```python
from build123d import *

# Parameters (mm, degrees)
SKETCH_1_R               = 275
SKETCH_1_R_2             = 255
EXTRUDE_1_DEPTH          = 10
EXTRUDE_2_DEPTH          = 10
SKETCH_8_R               = 2.65
SKETCH_8_R_2             = 1.65
SKETCH_8_R_3             = 2.15
CUT_EXTRUDE_1_DEPTH      = 21
SKETCH_9_OUTSIDE_W       = 707.614
SKETCH_9_OUTSIDE_H       = 707.614
CUT_EXTRUDE_2_DEPTH      = 21
EXTRUDE_3_DEPTH          = 10
SKETCH_11_W              = 11
SKETCH_11_H              = 6
CUT_EXTRUDE_3_DEPTH      = 509.636319812
CUT_EXTRUDE_3_DEPTH_BACK = 255.723154156
SKETCH_12_W              = 684.820669576
SKETCH_12_H              = 20
CUT_EXTRUDE_4_DEPTH      = 230.939436413
CUT_EXTRUDE_4_DEPTH_BACK = 534.420037555
SKETCH_14_R              = 4
CUT_EXTRUDE_6_DEPTH      = 11


with BuildPart() as part:
    # 草图1 → 凸台-拉伸1 (new body)
    with BuildSketch(Plane(origin=(0, 0, 0), x_dir=(1, 0, 0), z_dir=(0, 1, 0))):
        Circle(SKETCH_1_R)
        Circle(SKETCH_1_R_2, mode=Mode.SUBTRACT)
    extrude(amount=EXTRUDE_1_DEPTH)

    # 草图12 → 切除-拉伸4 (cut, two sides)
    with BuildSketch(Plane(origin=(84.710658728, 0, -125.893697679), x_dir=(-0.829665535, 0, -0.558260781), z_dir=(0.558260781, 0, -0.829665535))) as cut_extrude_4_sk:
        Rectangle(SKETCH_12_W, SKETCH_12_H)
    extrude(amount=CUT_EXTRUDE_4_DEPTH, mode=Mode.SUBTRACT)
    extrude(cut_extrude_4_sk.sketch, amount=-CUT_EXTRUDE_4_DEPTH_BACK, mode=Mode.SUBTRACT)


with BuildPart() as body_2:
    # 草图2 → 凸台-拉伸2 (new body)
    with BuildSketch(Plane(origin=(0, 10, 0), x_dir=(1, 0, 0), z_dir=(0, 1, 0))):
        with BuildLine():
            Line((-110.525139894, 257.262887824), (-25.423255477, 200))
            Line((-25.423255477, 200), (0, 200))
            Line((0, 200), (25.423255477, 200))
            Line((25.423255477, 200), (110.525139894, 257.262887824))
            ThreePointArc((110.525139894, 257.262887824), (197.989898732, 197.989898732), (257.262887824, 110.525139894))
            Line((257.262887824, 110.525139894), (200, 25.423255477))
            Line((200, 25.423255477), (200, 0))
            Line((200, 0), (200, -25.423255477))
            Line((200, -25.423255477), (257.262887824, -110.525139894))
            ThreePointArc((257.262887824, -110.525139894), (197.989898732, -197.989898732), (110.525139894, -257.262887824))
            Line((110.525139894, -257.262887824), (25.423255477, -200))
            Line((25.423255477, -200), (0, -200))
            Line((0, -200), (-25.423255477, -200))
            Line((-25.423255477, -200), (-110.525139894, -257.262887824))
            ThreePointArc((-110.525139894, -257.262887824), (-197.989898732, -197.989898732), (-257.262887824, -110.525139894))
            Line((-257.262887824, -110.525139894), (-200, -25.423255477))
            Line((-200, -25.423255477), (-200, 25.423255477))
            Line((-200, 25.423255477), (-257.262887824, 110.525139894))
            ThreePointArc((-257.262887824, 110.525139894), (-197.989898732, 197.989898732), (-110.525139894, 257.262887824))
        make_face()
        with BuildLine():
            Line((0, 185), (30, 185))
            Line((30, 185), (111.993839361, 240.171563565))
            ThreePointArc((111.993839361, 240.171563565), (187.383297014, 187.383297014), (240.171563565, 111.993839361))
            Line((240.171563565, 111.993839361), (185, 30))
            Line((185, 30), (185, 0))
            Line((185, 0), (185, -30))
            Line((185, -30), (240.171563565, -111.993839361))
            ThreePointArc((240.171563565, -111.993839361), (187.383297014, -187.383297014), (111.993839361, -240.171563565))
            Line((111.993839361, -240.171563565), (30, -185))
            Line((30, -185), (0, -185))
            Line((0, -185), (-30, -185))
            Line((-30, -185), (-111.993839361, -240.171563565))
            ThreePointArc((-111.993839361, -240.171563565), (-187.383297014, -187.383297014), (-240.171563565, -111.993839361))
            Line((-240.171563565, -111.993839361), (-185, -30))
            Line((-185, -30), (-185, 30))
            Line((-185, 30), (-240.171563565, 111.993839361))
            ThreePointArc((-240.171563565, 111.993839361), (-187.383297014, 187.383297014), (-111.993839361, 240.171563565))
            Line((-111.993839361, 240.171563565), (-30, 185))
            Line((-30, 185), (0, 185))
        make_face(mode=Mode.SUBTRACT)
    extrude(amount=EXTRUDE_2_DEPTH)

    # 草图8 → 切除-拉伸1 (cut, through all)
    with BuildSketch(Plane(origin=(0, 20, 0), x_dir=(1, 0, 0), z_dir=(0, 1, 0))):
        with Locations((-10, 192.5)):
            Circle(SKETCH_8_R)
        with Locations((10, 192.5)):
            Circle(SKETCH_8_R)
        with Locations((-10, -192.5)):
            Circle(SKETCH_8_R)
        with Locations((10, -192.5)):
            Circle(SKETCH_8_R)
        with Locations((192.5, 10)):
            Circle(SKETCH_8_R)
        with Locations((192.5, -10)):
            Circle(SKETCH_8_R)
        with Locations((-192.5, 10)):
            Circle(SKETCH_8_R)
        with Locations((-192.5, -10)):
            Circle(SKETCH_8_R)
        with Locations((-110.525139894, 248.223100485)):
            Circle(SKETCH_8_R_2)
        with Locations((-27.711627738, 192.5)):
            Circle(SKETCH_8_R)
        with Locations((-56.749921469, 212.03912734)):
            Circle(SKETCH_8_R)
        with Locations((-69.194904497, 220.413039057)):
            Circle(SKETCH_8_R)
        with Locations((-81.639887524, 228.786950774)):
            Circle(SKETCH_8_R)
        with Locations((-143.808163456, 231.45377032)):
            Circle(SKETCH_8_R_3)
        with Locations((-164.415519771, 217.299729706)):
            Circle(SKETCH_8_R_3)
        with Locations((-183.638937552, 201.316607082)):
            Circle(SKETCH_8_R_3)
        with Locations((-201.316607082, 183.638937552)):
            Circle(SKETCH_8_R_3)
        with Locations((-217.299729706, 164.415519771)):
            Circle(SKETCH_8_R_3)
        with Locations((-231.45377032, 143.808163456)):
            Circle(SKETCH_8_R_3)
        with Locations((-128.811575358, 240.123330241)):
            Circle(SKETCH_8_R)
        with Locations((-240.123330241, 128.811575358)):
            Circle(SKETCH_8_R)
        with Locations((-228.786950774, 81.639887524)):
            Circle(SKETCH_8_R)
        with Locations((-220.413039057, 69.194904497)):
            Circle(SKETCH_8_R)
        with Locations((-212.03912734, 56.749921469)):
            Circle(SKETCH_8_R)
        with Locations((-203.665215623, 44.304938442)):
            Circle(SKETCH_8_R)
        with Locations((-192.5, 27.711627738)):
            Circle(SKETCH_8_R)
        with Locations((-248.223100485, 110.525139894)):
            Circle(SKETCH_8_R_2)
        with Locations((192.5, 27.711627738)):
            Circle(SKETCH_8_R)
        with Locations((248.223100485, 110.525139894)):
            Circle(SKETCH_8_R_2)
        with Locations((203.665215623, 44.304938442)):
            Circle(SKETCH_8_R)
        with Locations((212.03912734, 56.749921469)):
            Circle(SKETCH_8_R)
        with Locations((220.413039057, 69.194904497)):
            Circle(SKETCH_8_R)
        with Locations((228.786950774, 81.639887524)):
            Circle(SKETCH_8_R)
        with Locations((240.123330241, 128.811575358)):
            Circle(SKETCH_8_R)
        with Locations((231.45377032, 143.808163456)):
            Circle(SKETCH_8_R_3)
        with Locations((128.811575358, 240.123330241)):
            Circle(SKETCH_8_R)
        with Locations((201.316607082, 183.638937552)):
            Circle(SKETCH_8_R_3)
        with Locations((183.638937552, 201.316607082)):
            Circle(SKETCH_8_R_3)
        with Locations((164.415519771, 217.299729706)):
            Circle(SKETCH_8_R_3)
        with Locations((143.808163456, 231.45377032)):
            Circle(SKETCH_8_R_3)
        with Locations((81.639887524, 228.786950774)):
            Circle(SKETCH_8_R)
        with Locations((69.194904497, 220.413039057)):
            Circle(SKETCH_8_R)
        with Locations((56.749921469, 212.03912734)):
            Circle(SKETCH_8_R)
        with Locations((110.525139894, 248.223100485)):
            Circle(SKETCH_8_R_2)
        with Locations((27.711627738, 192.5)):
            Circle(SKETCH_8_R)
        with Locations((217.299729706, 164.415519771)):
            Circle(SKETCH_8_R_3)
    extrude(amount=-CUT_EXTRUDE_1_DEPTH, mode=Mode.SUBTRACT)

    # 草图9 outside → 切除-拉伸2 (cut, through all)
    with BuildSketch(Plane(origin=(0, 20, 0), x_dir=(1, 0, 0), z_dir=(0, 1, 0))):
        Rectangle(SKETCH_9_OUTSIDE_W, SKETCH_9_OUTSIDE_H)
        Polygon((-28.994754224, 184.323595752), (-20.620842507, 196.76857878), (-83.675423179, 239.196398147), (-92.049334896, 226.751415119), align=None, mode=Mode.SUBTRACT)
    extrude(amount=-CUT_EXTRUDE_2_DEPTH, mode=Mode.SUBTRACT)

    # 草图10 → 凸台-拉伸3 (add)
    with BuildSketch(Plane(origin=(0, 20, 0), x_dir=(1, 0, 0), z_dir=(0, 1, 0))):
        Polygon((-28.539619055, 185), (-28.994754224, 184.323595752), (-30, 185), align=None)
    extrude(amount=-EXTRUDE_3_DEPTH)

    # 草图11 → 切除-拉伸3 (cut, two sides)
    with BuildSketch(Plane(origin=(-105.331501234, 0, -70.874881101), x_dir=(0.558260781, 0, -0.829665535), z_dir=(0.829665535, 0, 0.558260781))) as cut_extrude_3_sk:
        with Locations((144.240300571, 15)):
            Rectangle(SKETCH_11_W, SKETCH_11_H)
    extrude(amount=CUT_EXTRUDE_3_DEPTH, mode=Mode.SUBTRACT)
    extrude(cut_extrude_3_sk.sketch, amount=-CUT_EXTRUDE_3_DEPTH_BACK, mode=Mode.SUBTRACT)

    # 草图14 → 切除-拉伸6 (cut, through all)
    with BuildSketch(Plane.XZ.offset(-10)):
        with Locations((-47.5, -205.5)):
            Circle(SKETCH_14_R)
    extrude(amount=-CUT_EXTRUDE_6_DEPTH, mode=Mode.SUBTRACT)


solid = body_2.part
```
Input: part model. Units: mm. Frame: model coordinates. A direction names the side the tool comes from. Give positions to 0.01 mm unless a question says otherwise; leave off trailing zeros. Loops run counter-clockwise (first coordinate to the right, second up) from the corner with the lowest first, then second, coordinate; pieces in that order, holes last.
1) Section query C-C on x = -46. Return the cut outline in (y, z).
A:
outline: (10, -213.85) - (20, -213.85) - (20, -209.21) - (18, -209.21) - (18, -211.43) - (12, -211.43) - (12, -209.21) - (10, -209.21) - close; (10, -201.79) - (12, -201.79) - (12, -198.18) - (18, -198.18) - (18, -201.79) - (20, -201.79) - (20, -195.77) - (10, -195.77) - close
2) Section query D-D on z = -205.5. Return the cut outline in (x, y).
A:
outline: (-60.47, 10) - (-51.5, 10) - (-51.5, 12) - (-56.88, 12) - (-56.88, 18) - (-51.5, 18) - (-51.5, 20) - (-60.47, 20) - close; (-43.5, 10) - (-33.6, 10) - (-33.6, 20) - (-43.5, 20) - (-43.5, 18) - (-37.18, 18) - (-37.18, 12) - (-43.5, 12) - close
3) Section query B-B on z = -192.5. Return the cut outline in (x, y).
A:
outline: (-41.15, 10) - (-30.36, 10) - (-30.36, 12) - (-37.56, 12) - (-37.56, 18) - (-30.36, 18) - (-30.36, 20) - (-41.15, 20) - close; (-25.06, 10) - (-23.49, 10) - (-23.49, 12) - (-25.06, 12) - close; (-25.06, 18) - (-23.49, 18) - (-23.49, 20) - (-25.06, 20) - close
4) Mould query, pull axis X, two halves, no side actions, for faces 3 (the flat face through (-59, 20, -210)), 4 (the flat face through (-87.804, 11.737, -233.061)), 5 (the flat face through (-57, 12, -209)). Classes: released by +X, released by -X, zero draft, split by the parting line, or undercut.
A:
face 3: zero draft
face 4: released by -X
face 5: undercut
5) Contact query for flat-ended pins moving along their axis: pin 1 (5 mm diameter, centred on y = 14.5, z = -219, fed in from -X); pin 2 (3 mm diameter, centred on y = 16, z = -214, fed in from -X); pin 3 (2 mm diameter, centred on y = 11, z = -201.5, fed in from +X). Output: stop coordinate, or through.
A:
pin 1: stops at x = -84.24
pin 2: stops at x = -75.33
pin 3: stops at x = -26.17
6) Reachability of faces 1 (the flat face through (-59, 10, -210)), 2 (the flat face through (-52.823, 14.958, -216.026)) from +Z, -Z, +X, -X, +Y, -Y: full face, straight path, thin tool, end or side. Return the list, or none.
A:
face 1: +Z, -Z, +X, -X, -Y
face 2: none
7) Line query: L1, parallel to Y at x = -81, z = -223.5; L2, parallel to Z at x = -70.5, y = 13.75; L3, parallel to X at y = 14.5, z = -222.5. Output: solid intervals per line, ascending.
A:
L1: y = 10 to 12, 18 to 20
L2: z = -230.33 to -227.92, -214.66 to -212.25
L3: x = -85.73 to -82.15, -62.44 to -58.86
8) Section query A-A on y = 14.25. Return the cut outline in (x, z).
A:
outline: (-92.05, -226.75) - (-90.93, -228.41) - (-27.88, -185.98) - (-28.99, -184.32) - close; (-84.79, -237.54) - (-83.68, -239.2) - (-20.62, -196.77) - (-21.74, -195.11) - close
